Verification items for the finished model (mm, model axes). Face numbers are marked on the shaded views. A direction names the side the tool comes from. Round coordinates to 2 decimals unless told otherwise and drop trailing zeros. Loops run counter-clockwise (first coordinate to the right, second up) from the corner with the lowest first, then second, coordinate; pieces in that order, holes last. Notation, with made-up numbers: M -13.75,29 L 18.25,29 A4 cw 18.25,33 Z; hole C -13.75,12 d2. An arc over 180 degrees is marked long. Answer as CSV lines item,"result".
```python
from build123d import *

# Parameters (mm, degrees)
SKETCH_2_R               = 5.25
EXTRUDE_1_DEPTH          = 20
PATTERN_CIRCULAR_1_COUNT = 3
SKETCH_7_W               = 25
SKETCH_7_H               = 12
CUT_EXTRUDE_1_DEPTH      = 20
FILLET_1_R               = 1
SKETCH_9_W               = 7.609655
SKETCH_9_H               = 12
CUT_EXTRUDE_2_DEPTH      = 20
HOLE_WIZARD_M3_1_D       = 2.5
HOLE_WIZARD_M5_1_D       = 4.2
HOLE_WIZARD_M5_1_DEPTH   = 10
HOLE_WIZARD_M5_1_TIP     = 1.2618073


with BuildPart() as part:
    # 草图1 → 旋转1 (revolve)
    with BuildSketch(Plane(origin=(0, 0, 0), x_dir=(0, 0, -1), z_dir=(1, 0, 0)), mode=Mode.PRIVATE) as revolve_1_sk:
        Polygon((0, 0), (-30, 0), (-30, 13.061610641), (-35.8, 13.061610641), (-35.8, 63.5), (0, 63.5), align=None)
    revolve(revolve_1_sk.sketch.rotate(Axis((0, 0, 0), (0, 1, 0)), 180), axis=Axis((0, 0, 0), (0, 1, 0)))

    # 草图2 → 凸台-拉伸1 (add)
    with BuildSketch(Plane(origin=(0, 63.5, 0), x_dir=(1, 0, 0), z_dir=(0, 1, 0))):
        with Locations(Location((0, 0, 0), (0, 0, 90))):
            Circle(SKETCH_2_R)
    extrude(amount=EXTRUDE_1_DEPTH)

    # 草图3 → M4 螺纹孔1 (revolve, cut)
    with BuildSketch(Plane(origin=(0, 63.5, -20), x_dir=(0, 0, 1), z_dir=(1, 0, 0))):
        Polygon((0, 0), (0, 4.991420021), (1.65, 4), (1.65, 0), align=None)
    hole_wizard_m4_1 = revolve(axis=Axis((0, 69.85, -20), (0, -1, 0)), mode=Mode.SUBTRACT)

    # 草图5 → M1.2x0.25 螺纹孔1 (revolve, cut)
    with BuildSketch(Plane(origin=(0, 63.5, -7.8), x_dir=(0, 0, 1), z_dir=(1, 0, 0))):
        Polygon((0, 0), (0, 3.435408794), (0.475, 3.15), (0.475, 0), align=None)
    m1_2x0_25_1 = revolve(axis=Axis((0, 69.85, -7.8), (0, -1, 0)), mode=Mode.SUBTRACT)

    # 阵列(圆周)1: M4 螺纹孔1, M1.2x0.25 螺纹孔1 ×3 about axis
    pattern_circular_1_axis = Axis((0, 0, 0), (0, 1, 0))
    add([hole_wizard_m4_1.rotate(pattern_circular_1_axis, i * 360 / PATTERN_CIRCULAR_1_COUNT) for i in range(1, PATTERN_CIRCULAR_1_COUNT)], mode=Mode.SUBTRACT)
    add([m1_2x0_25_1.rotate(pattern_circular_1_axis, i * 360 / PATTERN_CIRCULAR_1_COUNT) for i in range(1, PATTERN_CIRCULAR_1_COUNT)], mode=Mode.SUBTRACT)

    # 草图7 → 切除-拉伸1 (cut)
    with BuildSketch(Plane.XY.offset(40)):
        with Locations((0, 7.061610641)):
            Rectangle(SKETCH_7_W, SKETCH_7_H)
    extrude(amount=-CUT_EXTRUDE_1_DEPTH, mode=Mode.SUBTRACT)

    # 圆角1
    fillet_1_edges = [part.edges().sort_by_distance(p)[0] for p in [
        (0, 83.5, 5.25),
    ]]
    fillet(fillet_1_edges, radius=FILLET_1_R)

    # 草图9 → 切除-拉伸2 (cut)
    with BuildSketch(Plane.XY.offset(4.25)):
        with Locations((0, 77.5)):
            Rectangle(SKETCH_9_W, SKETCH_9_H)
    extrude(amount=CUT_EXTRUDE_2_DEPTH, mode=Mode.SUBTRACT)

    # M3 螺纹孔1 (through all)
    with Locations(Plane.XY.offset(4.25)):
        with Locations((0, 80.5)):
            Hole(HOLE_WIZARD_M3_1_D / 2)

    # M5 螺纹孔1
    with Locations(Plane(origin=(0, 83.5, 0), x_dir=(1, 0, 0), z_dir=(0, 1, 0))):
        with Locations((0, 0)):
            Hole(HOLE_WIZARD_M5_1_D / 2, depth=HOLE_WIZARD_M5_1_DEPTH)
            with Locations((0, 0, -(HOLE_WIZARD_M5_1_DEPTH + HOLE_WIZARD_M5_1_TIP / 2))):  # 118° drill point
                Cone(0, HOLE_WIZARD_M5_1_D / 2, HOLE_WIZARD_M5_1_TIP, mode=Mode.SUBTRACT)


solid = part.part
```
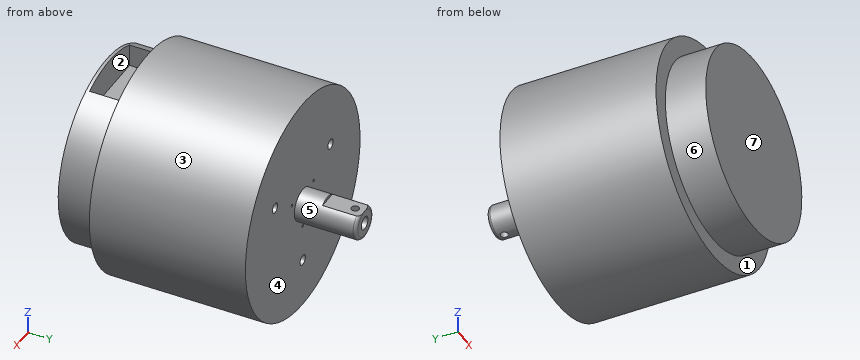
1) Draft check along Y on the marked faces 1, 2, 3 and 4. Enter one of: +Y half, -Y half, draft (parallel to the pull), parting line (faces both ways), or undercut.
Here are the results:
face 1,"undercut"
face 2,"undercut"
face 3,"draft"
face 4,"+Y half"
2) Section check A-A (y = 80.5). Record the cut outline in (x, z).
Here are the results:
outline,"M -3.08,4.25 A5.25 ccw -1.25,-5.1 L -1.25,-1.69 A2.1 cw -1.25,1.69 L -1.25,4.25 Z; M 1.25,-5.1 A5.25 ccw 3.08,4.25 L 1.25,4.25 L 1.25,1.69 A2.1 cw 1.25,-1.69 Z"
3) Set-up check for the marked faces 5, 6 and 7: record each of +Z, -Z, +X, -X, +Y, -Y from which the full face is reachable in a straight line by a thin tool's end or side.
Here are the results:
face 5,"+Y"
face 6,"-Y"
face 7,"+Z, -Z, +X, -X, -Y"
4) Section check C-C (z = -12). Record the cut outline in (x, y), plus the area to 3 significant figures.
Here are the results:
outline,"M -33.73,13.06 L -27.5,13.06 L -27.5,0 L 27.5,0 L 27.5,13.06 L 33.73,13.06 L 33.73,63.5 L -33.73,63.5 Z"
area,"4,120 mm^2"
5) Material ranges on probe 1 along X at (y, z) = (61, 10) (1 decimal); probe 2 along X at (y, z) = (61.45, 3.9); probe 3 along Y at (x, z) = (15.5, -8), recorded low to high.
Here are the results:
probe 1,"x = -34.4 to -19, -15.7 to 15.7, 19 to 34.4"
probe 2,"x = -35.59 to -7.23, -6.28 to 6.28, 7.23 to 35.59"
probe 3,"y = 0 to 63.5"
6) Section check D-D (x = 27). Record the cut outline in (y, z).
Here are the results:
outline,"M 0,-13.08 L 13.06,-13.08 L 13.06,-23.51 L 63.5,-23.51 L 63.5,23.51 L 13.06,23.51 L 13.06,13.08 L 0,13.08 Z"
7) Go/stop test with flat-tipped pins: pin 1 (1 mm diameter, centred on x = 11.5, y = 31, fed in from -Z); pin 2 (8 mm diameter, centred on y = 46.5, z = -4, fed in from +X); pin 3 (3 mm diameter, centred on y = 16.5, z = 12.5, fed in from -X); pin 4 (5 mm diameter, centred on x = 23.5, y = 68, fed in from +Z). Record where each tip stops, or that it passes through.
Here are the results:
pin 1,"stops at z = -34.07"
pin 2,"stops at x = 35.8"
pin 3,"stops at x = -34.07"
pin 4,"passes through"
8) Section check B-B (y = 62). State how many separate pieces and enclosed holes the cut face has, plus the area to 3 significant figures.
Here are the results:
separate pieces,"1"
enclosed holes,"6"
area,"4,000 mm^2"
